Source: CAD feature listing. Evaluate the final solid. Frame: model axes, mm. Face numbers are marked on the shaded views. A direction names the side the tool comes from. Give positions to 0.01 mm unless a question says otherwise; leave off trailing zeros. Write each loop counter-clockwise with the first axis right and the second up, starting at its lowest first coordinate (ties: lowest second). Pieces come first, ordered by that corner, then holes. Notation, with made-up numbers: (75, 6) -> (96, 6) arc R16 ccw to (96, 13) -> close; hole circle Ø5 at (75, 38). An arc over 180 degrees is marked (long way). Write item = value, one per line.
Solid Edge part; units mm, degrees
sketch "Sketch1" plane through (0, 0, 0) normal (0, -1, 0) x (1, 0, 0)
  line L0 (-24.05, 16.825) -> (-24.05, 15.5)
  line L1 (-24.05, 15.5) -> (-32.318, 15.5)
  line L2 (-32.318, 15.5) -> (-24.018, 7.2)
  line L3 (-24.018, 7.2) -> (-15.982, 7.2)
  line L4 (-15.982, 7.2) -> (-7.682, 15.5)
  line L5 (-7.682, 15.5) -> (-15.95, 15.5)
  line L6 (-15.95, 15.5) -> (-15.95, 16.825)
  arc A0 (-12.775, 20) -> (-15.95, 16.825) centre (-12.775, 16.825) ccw
  line L7 (-12.775, 20) -> (12.775, 20)
  arc A1 (15.95, 16.825) -> (12.775, 20) centre (12.775, 16.825) ccw
  line L8 (15.95, 16.825) -> (15.95, 15.5)
  line L9 (15.95, 15.5) -> (7.682, 15.5)
  line L10 (7.682, 15.5) -> (15.982, 7.2)
  line L11 (15.982, 7.2) -> (24.018, 7.2)
  line L12 (24.018, 7.2) -> (32.318, 15.5)
  line L13 (32.318, 15.5) -> (24.05, 15.5)
  line L14 (24.05, 15.5) -> (24.05, 16.825)
  arc A2 (27.225, 20) -> (24.05, 16.825) centre (27.225, 16.825) ccw
  line L15 (27.225, 20) -> (36.825, 20)
  arc A3 (40, 16.825) -> (36.825, 20) centre (36.825, 16.825) ccw
  line L16 (40, 16.825) -> (40, 7.225)
  arc A4 (36.825, 4.05) -> (40, 7.225) centre (36.825, 7.225) ccw
  line L17 (36.825, 4.05) -> (35.5, 4.05)
  line L18 (35.5, 4.05) -> (35.5, 12.318)
  line L19 (35.5, 12.318) -> (27.2, 4.018)
  line L20 (27.2, 4.018) -> (27.2, -4.018)
  line L21 (27.2, -4.018) -> (35.5, -12.318)
  line L22 (35.5, -12.318) -> (35.5, -4.05)
  line L23 (35.5, -4.05) -> (36.825, -4.05)
  arc A5 (40, -7.225) -> (36.825, -4.05) centre (36.825, -7.225) ccw
  line L24 (40, -7.225) -> (40, -16.825)
  arc A6 (36.825, -20) -> (40, -16.825) centre (36.825, -16.825) ccw
  line L25 (36.825, -20) -> (27.2248, -20)
  arc A7 (24.0498, -16.825) -> (27.2248, -20) centre (27.2248, -16.825) ccw
  line L26 (24.0498, -16.825) -> (24.0498, -15.5)
  line L27 (24.0498, -15.5) -> (32.318, -15.5)
  line L28 (32.318, -15.5) -> (24.018, -7.2)
  line L29 (24.018, -7.2) -> (15.982, -7.2)
  line L30 (15.982, -7.2) -> (7.682, -15.5)
  line L31 (7.682, -15.5) -> (15.9498, -15.5)
  line L32 (15.9498, -15.5) -> (15.9498, -16.825)
  arc A8 (12.7748, -20) -> (15.9498, -16.825) centre (12.7748, -16.825) ccw
  line L33 (12.7748, -20) -> (-12.775, -20)
  arc A9 (-15.95, -16.825) -> (-12.775, -20) centre (-12.775, -16.825) ccw
  line L34 (-15.95, -16.825) -> (-15.95, -15.5)
  line L35 (-15.95, -15.5) -> (-7.682, -15.5)
  line L36 (-7.682, -15.5) -> (-15.982, -7.2)
  line L37 (-15.982, -7.2) -> (-24.018, -7.2)
  line L38 (-24.018, -7.2) -> (-32.318, -15.5)
  line L39 (-32.318, -15.5) -> (-24.05, -15.5)
  line L40 (-24.05, -15.5) -> (-24.05, -16.825)
  arc A10 (-27.225, -20) -> (-24.05, -16.825) centre (-27.225, -16.825) ccw
  line L41 (-27.225, -20) -> (-36.825, -20)
  arc A11 (-40, -16.825) -> (-36.825, -20) centre (-36.825, -16.825) ccw
  line L42 (-40, -16.825) -> (-40, -7.2248)
  arc A12 (-36.825, -4.0498) -> (-40, -7.2248) centre (-36.825, -7.2248) ccw
  line L43 (-36.825, -4.0498) -> (-35.5, -4.0498)
  line L44 (-35.5, -4.0498) -> (-35.5, -12.318)
  line L45 (-35.5, -12.318) -> (-27.2, -4.018)
  line L46 (-27.2, -4.018) -> (-27.2, 4.018)
  line L47 (-27.2, 4.018) -> (-35.5, 12.318)
  line L48 (-35.5, 12.318) -> (-35.5, 4.0502)
  line L49 (-35.5, 4.0502) -> (-36.825, 4.0502)
  arc A13 (-40, 7.2252) -> (-36.825, 4.0502) centre (-36.825, 7.2252) ccw
  line L50 (-40, 7.2252) -> (-40, 16.825)
  arc A14 (-36.825, 20) -> (-40, 16.825) centre (-36.825, 16.825) ccw
  line L51 (-36.825, 20) -> (-27.225, 20)
  arc A15 (-24.05, 16.825) -> (-27.225, 20) centre (-27.225, 16.825) ccw
  circle A16 centre (-20, 0) radius 3.683
  circle A17 centre (20, 0) radius 3.683
  line L52 (-4.5, 4.05) -> (4.5, 4.05)
  line L53 (4.5, 4.05) -> (4.5, 12.318)
  line L54 (4.5, 12.318) -> (12.8, 4.018)
  line L55 (12.8, 4.018) -> (12.8, -4.018)
  line L56 (12.8, -4.018) -> (4.5, -12.318)
  line L57 (4.5, -12.318) -> (4.5, -4.05)
  line L58 (4.5, -4.05) -> (-4.5, -4.05)
  line L59 (-4.5, -4.05) -> (-4.5, -12.318)
  line L60 (-4.5, -12.318) -> (-12.8, -4.018)
  line L61 (-12.8, -4.018) -> (-12.8, 4.018)
  line L62 (-12.8, 4.018) -> (-4.5, 12.318)
  line L63 (-4.5, 12.318) -> (-4.5, 4.05)
extrude "Protrusion1" add sketch "Sketch1" against normal blind 41.275
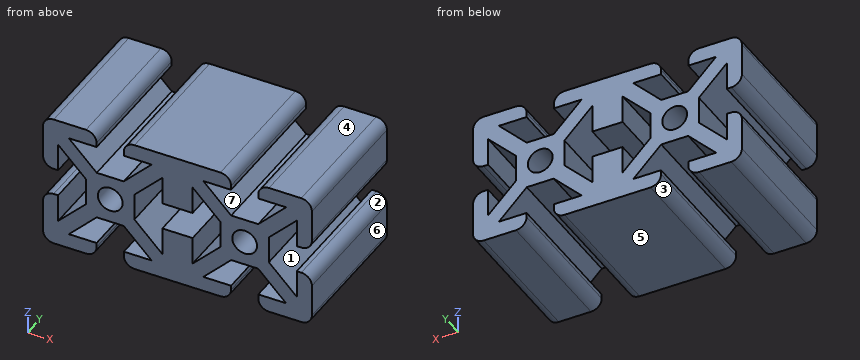
1) Cut plane D-D (y = 27.5). State how many separate pieces and enclosed holes the cut face has, then the cut area to 3 significant figures.
Computed:
separate_pieces = 1
enclosed_holes = 3
area = 1,700 mm²
2) Cut plane A-A (x = 3.5). Return the cut outline in (y, z) (3 decimals), then the cut area to 3 significant figures.
Computed:
outline = (0, -20) -> (41.275, -20) -> (41.275, -4.05) -> (0, -4.05) -> close; (0, 4.05) -> (41.275, 4.05) -> (41.275, 20) -> (0, 20) -> close
area = 1,320 mm²
3) Draft query along Z for the marked faces 5, 6 and 7. Return one class per face: pulls with the +Z half, pulls with the -Z half, needs draft (parallel to the pull), parting line crosses it, or undercut.
Computed:
face_5 = pulls with the -Z half
face_6 = needs draft
face_7 = undercut
4) Cut plane B-B (z = 0). Return the cut outline in (x, y) (3 decimals), then the cut area to 3 significant figures.
Computed:
outline = (-27.2, 0) -> (-23.683, 0) -> (-23.683, 41.275) -> (-27.2, 41.275) -> close; (-16.317, 0) -> (-12.8, 0) -> (-12.8, 41.275) -> (-16.317, 41.275) -> close; (12.8, 0) -> (16.317, 0) -> (16.317, 41.275) -> (12.8, 41.275) -> close; (23.683, 0) -> (27.2, 0) -> (27.2, 41.275) -> (23.683, 41.275) -> close
area = 581 mm²
5) Cut plane C-C (x = 26). Return the cut outline in (y, z) (3 decimals), then the cut area to 3 significant figures.
Computed:
outline = (0, -19.754) -> (41.275, -19.754) -> (41.275, -15.5) -> (0, -15.5) -> close; (0, -9.182) -> (41.275, -9.182) -> (41.275, 9.182) -> (0, 9.182) -> close; (0, 15.5) -> (41.275, 15.5) -> (41.275, 19.754) -> (0, 19.754) -> close
area = 1,110 mm²
6) Contact query for flat-ended pins moving along their axis: pin 1 (2 mm diameter, centred on x = -15, y = 9, fed in from -Z); pin 2 (2.5 mm diameter, centred on x = 18.5, y = 16.5, fed in from -Z); pin 3 (9 mm diameter, centred on y = 26.5, z = -0.5, fed in from +X). Output: stop coordinate, or through.
Computed:
pin_1 = -19.75
pin_2 = -7.2
pin_3 = 39.09
7) Material intervals for L1, parallel to X at y = 31, z = -14.5; L2, parallel to Z at x = 10.5, y = 32; L3, parallel to Z at x = -30, y = 39.5, sorted ascending.
Computed:
L1 = -40 to -31.32, -8.68 to 8.68, 31.32 to 40
L2 = -20 to -15.5, -12.68 to -6.32, 6.32 to 12.68, 15.5 to 20
L3 = -20 to -15.5, -13.18 to -6.82, 6.82 to 13.18, 15.5 to 20
8) Access query for the marked faces 1, 2, 3 and 4. Directions: +Z, -Z, +X, -X, +Y, -Y. A direction counts if a zero-diameter tool reaches every point of the face in a straight line with its end or side. Return the directions, or none.
Computed:
face_1 = +Y, -Y
face_2 = +X, +Y, -Y
face_3 = -Z, +Y, -Y
face_4 = +Z, +X, -X, +Y, -Y
